Source: CAD feature listing. Evaluate the final solid. Frame: model axes, mm. A direction names the side the tool comes from. Coordinates: 2 decimals unless noted, no trailing zeros. Write each loop counter-clockwise with the first axis right and the second up, starting at its lowest first coordinate (ties: lowest second). Pieces come first, ordered by that corner, then holes. Notation, with made-up numbers: (53.25, 24) -> (61.25, 24) arc R20 cw to (61.25, 41) -> close; hole circle Ø6 at (-24, -24.75). An arc over 180 degrees is marked (long way). One line per item, written item: value. Start each with the question number.
1. Section query C-C, the plane y = 0.95. Output: boundary loops of the cut face in (x, z).
2. Section query B-B, the plane z = 62.5. Output: boundary loops of the cut face in (x, y).
3. Mould query, pull axis X, two halves, no side actions, for faces 3 (the flat face through (-11.04, 2.96, 14.4)), 4 (the cylindrical face through (3.95, 2.958, 67.476)), 5 (the flat face through (21, 6, 24)). Classes: released by +X, released by -X, zero draft, split by the parting line, or undercut.
4. Line query: line 1 (X direction, y = 1.8, z = 62.5); line 2 (X direction, y = 3.45, z = 39.5); line 3 (Z direction, x = 9, y = 2.8). Output: solid intervals per line, ascending.
5. Section query A-A, the plane x = -6. Output: boundary loops of the cut face in (y, z).
6. Access query for faces 1 (the flat face through (-11.8, 3, 13.5)), 2 (the cylindrical face through (3.195, 2.958, -13.514)). Directions: +Z, -Z, +X, -X, +Y, -Y. A direction counts if a zero-diameter tool reaches every point of the face in a straight line with its end or side. Return the directions, or none.
7. First-contact query: P1, Ø10, axis at x = -10, z = 39, coming from the +Y side; P2, Ø1, axis at x = 14, y = 4.5, coming from the +Z side; P3, Ø1, axis at y = 3, z = 14.5, coming from the -X side; P4, Ø1.5, axis at x = 14.5, y = 5.5, coming from the +Z side. Flat tips, straight axial feed; report the tip coordinate or a pass-through.
Autodesk Inventor part; units mm, degrees
ref_plane "YZ Plane" through (0, 0, 0) normal (1, 0, 0) x (0, 1, 0)
ref_plane "XZ Plane" through (0, 0, 0) normal (0, 1, 0) x (-1, 0, 0)
ref_plane "XY Plane" through (0, 0, 0) normal (0, 0, 1) x (1, 0, 0)
sketch "Sketch1" plane through (0, 0, 0) normal (0, 1, 0) x (-1, 0, 0)
  arc A0 (18.3066, 36.6819) -> (-24.9519, 36.6819) centre (-3.3227, 43.7344) ccw
  arc A1 (-10.2155, -8.5131) -> (3.5702, -8.5131) centre (-3.3227, -6.2656) ccw
  line L0 (-24.9519, 36.6819) -> (-10.2155, -8.5131)
  line L1 (18.3066, 36.6819) -> (3.5702, -8.5131)
  line L2 (-25.9027, 36.3719) -> (-11.1663, -8.8231)
  arc A2 (-11.1663, -8.8231) -> (4.5209, -8.8231) centre (-3.3227, -6.2656) ccw
  line L3 (4.5209, -8.8231) -> (19.2573, 36.3719)
  arc A3 (19.2573, 36.3719) -> (-25.9027, 36.3719) centre (-3.3227, 43.7344) ccw
  point P0 (0, 0)
  dimension "d0" = 45.5
  dimension "d1" = 14.5
  dimension "d2" = 50
  dimension "d3" = 1
extrude "Extrusion1" add sketch "Sketch1" along normal blind 6
properties part number "COTS_Optibelt_Omega_HTD3M_204T_6mm"
Computed values:
1. outline: (-19.26, 36.37) -> (-4.52, -8.82) arc R8.25 ccw to (11.17, -8.82) -> (25.9, 36.37) arc R23.75 ccw (long way) to start; hole (-18.31, 36.68) -> (-3.57, -8.51) arc R7.25 ccw to (10.22, -8.51) -> (24.95, 36.68) arc R22.75 ccw (long way) to start
2. outline: (-11.23, 0) -> (-9.54, 0) -> (-9.54, 6) -> (-11.23, 6) -> close; (16.18, 0) -> (17.88, 0) -> (17.88, 6) -> (16.18, 6) -> close
3. face 3: undercut
3. face 4: split by the parting line
3. face 5: zero draft
4. line 1: x = -11.23 to -9.54, 16.18 to 17.88
4. line 2: x = -20.05 to -19.03, 25.68 to 26.69
4. line 3: z = -12.25 to -10.77, 65.76 to 66.8
5. outline: (0, -4.29) -> (6, -4.29) -> (6, -1.06) -> (0, -1.06) -> close; (0, 64.49) -> (6, 64.49) -> (6, 65.58) -> (0, 65.58) -> close
6. face 1: -Z, -X, +Y, -Y
6. face 2: +Y, -Y
7. P1: passes through
7. P2: stops at z = 65.19
7. P3: stops at x = -12.29
7. P4: stops at z = 65.07
